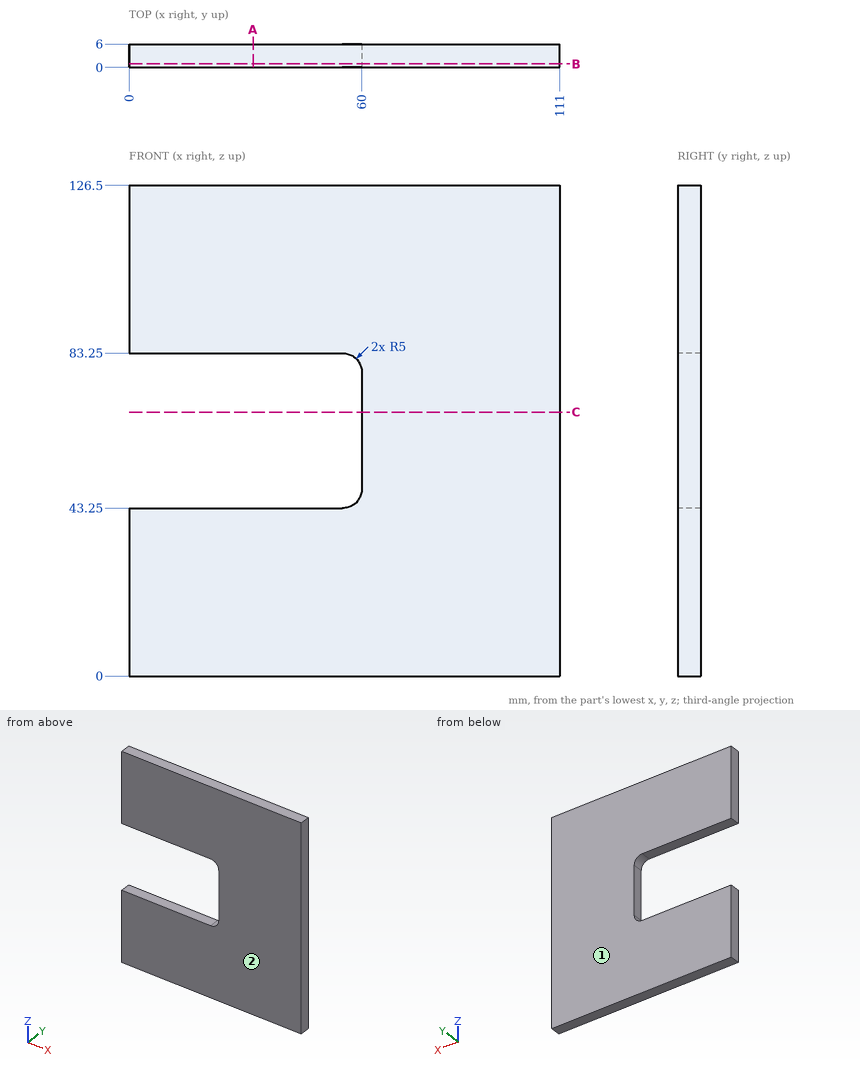
Answer from the drawing. Dimensions are ordinates in mm from the lowest x, y and z of the part. Give positions to 0.01 mm unless a question says otherwise; leave off trailing zeros. Loops run counter-clockwise (first coordinate to the right, second up) from the corner with the lowest first, then second, coordinate; pieces in that order, holes last.
Item 1: Find the intervals of material crossed by line 1 along Z through (x, y) = (55.5, 2.25); line 2 along Z through (x, y) = (39, 3.4); line 3 along X through (y, z) = (1.1, 73), in increasing order.
Item 2: The part is cut by section C-C (z = 68). Write down the section's boundary in (x, y).
Item 3: The part is cut by section A-A (x = 32). Write down the section's boundary in (y, z).
Item 4: The part is cut by section B-B (y = 0.9). Write down the section's boundary in (x, z), and give its area (3 significant figures).
Item 5: The mould has two halves that part along Y. Classify the marked faces 1 and 2: released by +Y, released by -Y, zero draft, split by the parting line, or undercut.
Taken from the geometry:
1. line 1: z = 0 to 43.28, 83.22 to 126.5
1. line 2: z = 0 to 43.25, 83.25 to 126.5
1. line 3: x = 60 to 111
2. outline: (60, 0) - (111, 0) - (111, 6) - (60, 6) - close
3. outline: (0, 0) - (6, 0) - (6, 43.25) - (0, 43.25) - close; (0, 83.25) - (6, 83.25) - (6, 126.5) - (0, 126.5) - close
4. outline: (0, 0) - (111, 0) - (111, 126.5) - (0, 126.5) - (0, 83.25) - (55, 83.25) arc R5 cw to (60, 78.25) - (60, 48.25) arc R5 cw to (55, 43.25) - (0, 43.25) - close
4. area: 11,700 mm2
5. face 1: released by +Y
5. face 2: released by -Y
